```python
from build123d import *

# Parameters (mm, degrees)
SKETCH_2_R = 4


with BuildPart() as part:
    # По траектории1: sweep along a path in Эскиз1
    with BuildLine(Plane(origin=(0, 0, 0), x_dir=(0, 0, -1), z_dir=(1, 0, 0))) as sweep_1_path:
        Line((0, -15), (35, -15))
        ThreePointArc((35, -15), (42.071067812, -12.071067812), (45, -5))
        Line((45, -5), (45, 5))
        ThreePointArc((45, 5), (42.071067812, 12.071067812), (35, 15))
        Line((35, 15), (0, 15))
    # Эскиз2 → По траектории1 (sweep)
    with BuildSketch(Plane.XY):
        with Locations((0, -15)):
            Circle(SKETCH_2_R)
    sweep(path=sweep_1_path.line)

    # Зеркальное отражение1: part across face


with BuildPart() as part_1:
    add(part.part)
    add(part.part.mirror(Plane(origin=(0, 15, 0), x_dir=(1, 0, 0), z_dir=(0, 0, 1))))


solid = part_1.part
```
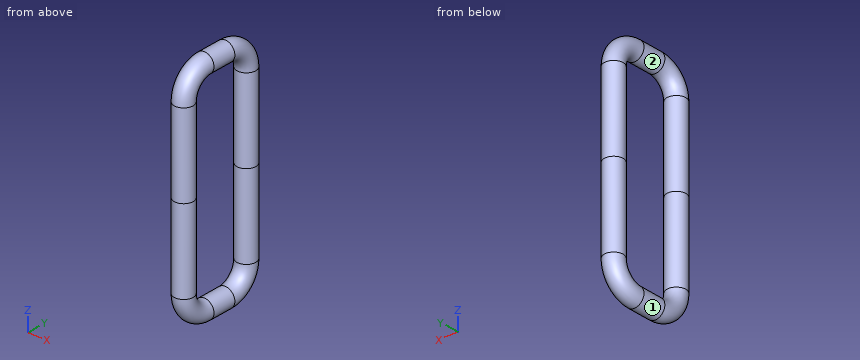
Could you check a few things on this model? Use its own coordinates, in mm. Face numbers are marked on the shaded views. Coordinates: 2 decimals unless noted, no trailing zeros. Order: outer loops, then holes, each group sorted by start corner. A loop starts at its lowest first (then second) coordinate and runs counter-clockwise, first axis right, second up. Notation, with made-up numbers: M 57.5,30.25 L 111.5,30.25 A26 ccw 111.5,51.25 Z; hole C 77.5,-30.5 d1. An arc over 180 degrees is marked long. Use one line per item in the form item = value. Start each with the question number.
1. Please list where these lines run through material, in increasing order: line 1 (Y direction, x = -0.75, z = -30); line 2 (Z direction, x = -3.5, y = -10); line 3 (Y direction, x = -3.5, z = 7.5).
2. Suppose I cut it at B-B on z = 14. Write out the boundary of the cut face in (x, y).
3. We'd pull the mould along Y, two halves only. Please class the marked faces 1 and 2: +Y half, -Y half, draft (parallel to the pull), parting line (faces both ways), or undercut.
4. Suppose I cut it at A-A on x = 0. Write out the boundary of the cut face in (y, z).
5. For pin 1 (10 mm diameter, centred on y = -3.5, z = -35, fed in from +X); pin 2 (4 mm diameter, centred on x = 3, z = -13, fed in from +Y); pin 3 (1.5 mm diameter, centred on x = -3, z = -25.5, fed in from -Y), each with a flat end and sliding along its axis, tell me the tip position at first contact or that it passes through.
Geometry says:
q1.line_1 = -18.93 to -11.07, 11.07 to 18.93
q1.line_2 = -45.84 to -41.33, 41.33 to 45.84
q1.line_3 = -16.94 to -13.06, 13.06 to 16.94
q2.outline = C 0,-15 d8; C 0,15 d8
q3.face_1 = undercut
q3.face_2 = undercut
q4.outline = M -19,-35 A14 ccw -5,-49 L 5,-49 A14 ccw 19,-35 L 19,35 A14 ccw 5,49 L -5,49 A14 ccw -19,35 Z; hole M -11,-35 A6 ccw -5,-41 L 5,-41 A6 ccw 11,-35 L 11,35 A6 ccw 5,41 L -5,41 A6 ccw -11,35 Z
q5.pin_1 = through
q5.pin_2 = 18.87
q5.pin_3 = -18.31
